from build123d import *

# Parameters (mm, degrees)
SKETCH1_R                 = 23
BOSS_EXTRUDE1_DEPTH       = 20
SKETCH2_R                 = 4
CUT_EXTRUDE1_DEPTH        = 20
M3X0_5_TAPPED_HOLE1_D     = 2.5
M3X0_5_TAPPED_HOLE1_DEPTH = 6.5
M3X0_5_TAPPED_HOLE1_TIP   = 0.751075774


with BuildPart() as part:
    # Sketch1 → Boss-Extrude1 (new body)
    with BuildSketch(Plane(origin=(0, 0, 0), x_dir=(1, 0, 0), z_dir=(0, 1, 0))):
        Circle(SKETCH1_R)
    extrude(amount=BOSS_EXTRUDE1_DEPTH)

    # Sketch2 → Cut-Extrude1 (cut)
    with BuildSketch(Plane(origin=(0, 20, 0), x_dir=(1, 0, 0), z_dir=(0, 1, 0))):
        Circle(SKETCH2_R)
    extrude(amount=-CUT_EXTRUDE1_DEPTH, mode=Mode.SUBTRACT)

    # M3x0.5 Tapped Hole1
    with Locations(Plane(origin=(0, 0, 0), x_dir=(-1, 0, 0), z_dir=(0, -1, 0))):
        with Locations((6.717514421, 6.717514421), (-7.5, 0), (7.5, 0), (0, 7.5), (0, -7.5), (-6.717514421, 6.717514421), (-6.717514421, -6.717514421), (6.717514421, -6.717514421)):
            Hole(M3X0_5_TAPPED_HOLE1_D / 2, depth=M3X0_5_TAPPED_HOLE1_DEPTH)
            with Locations((0, 0, -(M3X0_5_TAPPED_HOLE1_DEPTH + M3X0_5_TAPPED_HOLE1_TIP / 2))):  # 118° drill point
                Cone(0, M3X0_5_TAPPED_HOLE1_D / 2, M3X0_5_TAPPED_HOLE1_TIP, mode=Mode.SUBTRACT)


solid = part.part
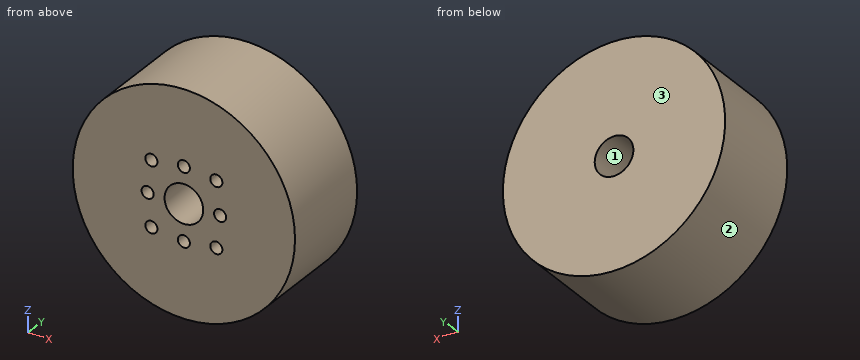
Design review of the part built by this model. Coordinates are the model's own, in mm. Face numbers are marked on the shaded views. Give positions to 0.01 mm unless a question says otherwise; leave off trailing zeros. Write each loop counter-clockwise with the first axis right and the second up, starting at its lowest first coordinate (ties: lowest second). Pieces come first, ordered by that corner, then holes. Notation, with made-up numbers: M 65,14.25 L 104,14.25 A19 ccw 104,40.25 Z; hole C 62.5,2 d3. An arc over 180 degrees is marked long. Answer as a JSON object with one key per item and string values. Group by question number.
1) Clearance check with flat-ended pins moving along their axes: pin 1 Ø5 at (x, z) = (0, 0) entering from -Y; pin 2 Ø6 at (y, z) = (6.5, 15) entering from -X; pin 3 Ø4 at (x, y) = (-10.5, 16.5) entering from -Z; pin 4 Ø2 at (x, z) = (6.72, -6.72) entering from -Y. State where each tip first meets the part, or that it passes through.
2) We need section B-B (y = 15.5). Give the boundary of the cut face in (x, z), and give its area (3 significant figures).
3) We need section C-C (y = 5.5). Count the separate pieces of the cut face and the enclosed holes in it, and give its area (3 significant figures).
4) Mouldability with a two-part tool opening along Z and no side actions: class the marked faces 1, 2 and 3 as released by +Z, released by -Z, zero draft, split by the parting line, or undercut.
5) We need section A-A (x = -2). Give the boundary of the cut face in (y, z).
6) For line 1 along Z through (x, y) = (0, 3); line 2 along Z through (x, y) = (6, 3.25); line 3 along X through (y, z) = (4.5, 7.5), list the stretches that pass through material, from the lowest coordinate up.
7) We need section D-D (z = -17). Give the boundary of the cut face in (x, y).
Answer key:
{
 "1": {"pin 1": "passes through", "pin 2": "stops at x = -19.62", "pin 3": "stops at z = -21.37", "pin 4": "stops at y = 6.65"},
 "2": {"outline": "C 0,0 d46; hole C 0,0 d8", "area": "1,610 mm²"},
 "3": {"separate pieces": "1", "enclosed holes": "9", "area": "1,570 mm²"},
 "4": {"face 1": "undercut", "face 2": "split by the parting line", "face 3": "zero draft"},
 "5": {"outline": "M 0,-22.91 L 20,-22.91 L 20,-3.46 L 0,-3.46 Z; M 0,3.46 L 20,3.46 L 20,22.91 L 0,22.91 Z"},
 "6": {"line 1": "z = -23 to -8.75, -6.25 to -4, 4 to 6.25, 8.75 to 23", "line 2": "z = -22.2 to -7.74, -5.69 to 5.69, 7.74 to 22.2", "line 3": "x = -21.74 to -7.69, -5.74 to -1.25, 1.25 to 5.74, 7.69 to 21.74"},
 "7": {"outline": "M -15.49,0 L 15.49,0 L 15.49,20 L -15.49,20 Z"}
}
